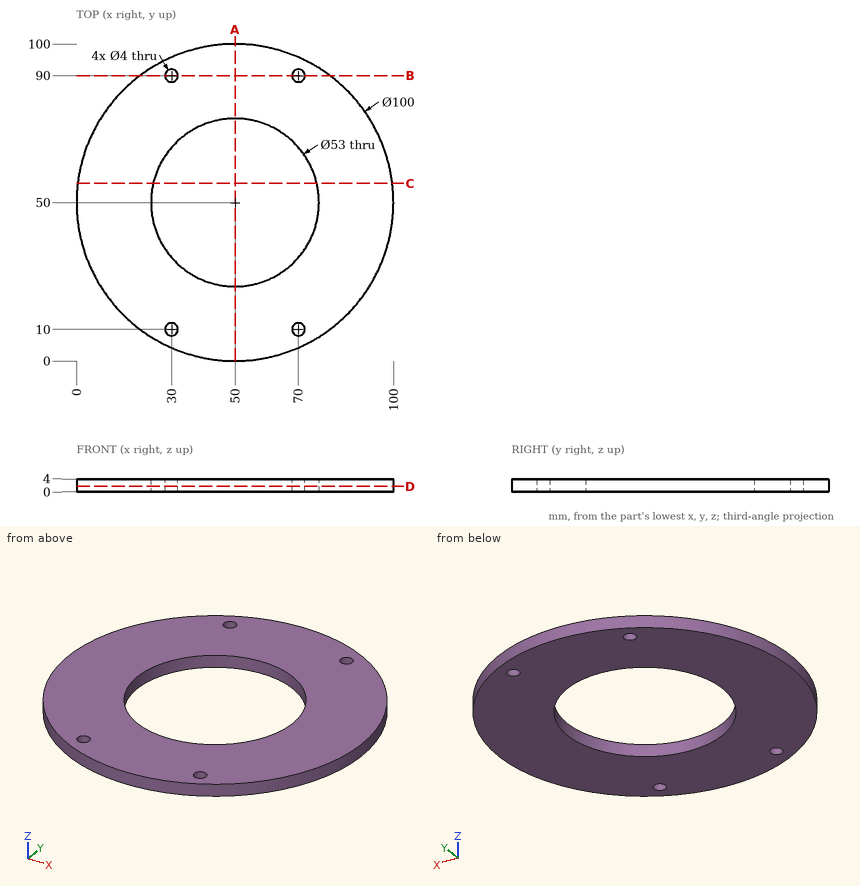
Can you work these out from the drawing? Everything is in mm from the part's minimum corner. Give positions to 0.01 mm unless a question says otherwise; leave off trailing zeros. Write each loop counter-clockwise with the first axis right and the second up, starting at its lowest first coordinate (ties: lowest second). Pieces come first, ordered by that corner, then holes. Notation, with made-up numbers: M 44.25,44.25 L 95.25,44.25 A16 ccw 95.25,53.25 Z; hole C -29,27.5 d6. An arc over 180 degrees is marked long. Answer in a Markdown table with one row per item. Add a question column.
Item 1: Please list where these lines run through material, in increasing order: L1, parallel to Y at x = 50, z = 1.7; L2, parallel to Y at x = 30, z = 1.55; L3, parallel to X at y = 52, z = 3.7.
Item 2: Imagine slicing it at A-A, the plane x = 50. Write out the boundary of the cut face in (y, z), plus the area to 3 significant figures.
Item 3: Imagine slicing it at C-C, the plane y = 56. Write out the boundary of the cut face in (x, z).
Item 4: For pin 1 Ø1.5 at (y, z) = (37, 1.5) entering from -X; pin 2 Ø1 at (y, z) = (73.5, 1.5) entering from -X; pin 3 Ø5 at (x, y) = (70, 10) entering from -Z, each with a flat end and sliding along its axis, tell me the tip position at first contact or that it passes through.
Item 5: Imagine slicing it at D-D, the plane z = 1.65. Write out the boundary of the cut face in (x, y), plus the area to 3 significant figures.
Item 6: Imagine slicing it at B-B, the plane y = 90. Write out the boundary of the cut face in (x, z).
Evaluation:
| question | item | result |
|---|---|---|
| 1 | L1 | y = 0 to 23.5, 76.5 to 100 |
| 1 | L2 | y = 4.17 to 8, 12 to 32.61, 67.39 to 88, 92 to 95.83 |
| 1 | L3 | x = 0.04 to 23.58, 76.42 to 99.96 |
| 2 | outline | M 0,0 L 23.5,0 L 23.5,4 L 0,4 Z; M 76.5,0 L 100,0 L 100,4 L 76.5,4 Z |
| 2 | area | 188 mm² |
| 3 | outline | M 0.36,0 L 24.19,0 L 24.19,4 L 0.36,4 Z; M 75.81,0 L 99.64,0 L 99.64,4 L 75.81,4 Z |
| 4 | pin 1 | stops at x = 1.52 |
| 4 | pin 2 | stops at x = 5.6 |
| 4 | pin 3 | stops at z = 0 |
| 5 | outline | C 50,50 d100; hole C 50,50 d53; hole C 30,10 d4; hole C 30,90 d4; hole C 70,10 d4; hole C 70,90 d4 |
| 5 | area | 5,600 mm² |
| 6 | outline | M 20,0 L 28,0 L 28,4 L 20,4 Z; M 32,0 L 68,0 L 68,4 L 32,4 Z; M 72,0 L 80,0 L 80,4 L 72,4 Z |
